Geometry: final body of the model. Coordinates: model frame, mm. Give positions to 0.01 mm unless a question says otherwise; leave off trailing zeros. Loops run counter-clockwise (first coordinate to the right, second up) from the corner with the lowest first, then second, coordinate; pieces in that order, holes last. Notation, with made-up numbers: (63.5, 65.5) - (91.5, 65.5) arc R26 cw to (91.5, 104.5) - close; hole circle Ø10 at (-3.75, 21.25). An arc over 180 degrees is marked (long way). Answer in a Markdown table with one row per item.
from build123d import *

# Parameters (mm, degrees)
F0_R     = 1.65
F0_R_2   = 2.55
F0_W     = 5
F0_H     = 10
F0_R_3   = 1.5
F0_R_4   = 3.555
F1_DEPTH = 4.75
F2_R     = 1
F3_DEPTH = 20
F4_R     = 3.555
F4_R_2   = 2.55
F5_DEPTH = 4.75


# Not quite as in the source:
# - ends of sketch curves that miss each other by under 0.0002 mm in the source are joined


with BuildPart() as f1:
    # F0 (on Top) → F1 (new body)
    with BuildSketch(Plane.XY):
        with BuildLine():
            Line((-47.640397, 42.115595), (-100.031737, 108.050449))
            ThreePointArc((-100.031737, 108.050449), (-107.8442155419, 109.1246397394), (-109.2715048598, 101.368896092))
            Line((-109.2715048598, 101.368896092), (-54.999977, 18.664241))
            Line((-54.999977, 18.664241), (-54.999977, -18.664242))
            Line((-54.999977, -18.664242), (-109.271505, -101.368897))
            ThreePointArc((-109.271505, -101.368897), (-107.8441644553, -109.1246766812), (-100.031658534, -108.0503513703))
            Line((-100.031658534, -108.0503513703), (-47.643302, -42.116283))
            ThreePointArc((-47.643302, -42.116283), (-33.7130803066, -30.9767526972), (-16.325566, -27))
            Line((-16.325566, -27), (16.325565, -27))
            ThreePointArc((16.325565, -27), (33.7130793066, -30.9767526972), (47.6433013924, -42.1162826882))
            Line((47.6433013924, -42.1162826882), (100.031658, -108.050351))
            ThreePointArc((100.031658, -108.050351), (107.8441644255, -109.1246767027), (109.2715050175, -101.3688963323))
            Line((109.2715050175, -101.3688963323), (54.999976, -18.664242))
            Line((54.999976, -18.664242), (54.999976, 18.664241))
            Line((54.999976, 18.664241), (109.271504, 101.368896))
            ThreePointArc((109.271504, 101.368896), (107.8442155121, 109.1246397609), (100.0317360662, 108.0504489474))
            Line((100.0317360662, 108.0504489474), (47.640396, 42.115595))
            ThreePointArc((47.640396, 42.115595), (33.7103248028, 30.9765618002), (16.323206, 27))
            Line((16.323206, 27), (-16.323206, 27))
            ThreePointArc((-16.323206, 27), (-33.710325083, 30.9765619354), (-47.640397, 42.115595))
        make_face()
        with Locations((-104.5, -104.5)):
            Circle(F0_R, mode=Mode.SUBTRACT)
        with Locations((-44.444977, -20.807752)):
            Circle(F0_R_2, mode=Mode.SUBTRACT)
        with Locations((-49.499977, 0)):
            Rectangle(F0_W, F0_H, mode=Mode.SUBTRACT)
        with BuildLine():
            Line((-19.581953, -16.373154), (-39.803759, -2.743263))
            ThreePointArc((-39.803759, -2.743263), (-40.6136447533, -1.8442487652), (-40.906473, -0.670199))
            Line((-40.906473, -0.670199), (-40.906473, 0.670176))
            ThreePointArc((-40.906473, 0.670176), (-40.6136450793, 1.8442251525), (-39.8037598701, 2.7432388072))
            Line((-39.8037598701, 2.7432388072), (-19.581955, 16.373149))
            ThreePointArc((-19.581955, 16.373149), (-17.0106188475, 16.5072580793), (-15.684668, 14.300086))
            Line((-15.684668, 14.300086), (-15.684668, -14.30009))
            ThreePointArc((-15.684668, -14.30009), (-17.0106178687, -16.5072615586), (-19.581953, -16.373154))
        make_face(mode=Mode.SUBTRACT)
        with Locations((-10, -10)):
            Circle(F0_R_3, mode=Mode.SUBTRACT)
        with Locations((104.5, -104.5)):
            Circle(F0_R, mode=Mode.SUBTRACT)
        with Locations((10, -10)):
            Circle(F0_R_3, mode=Mode.SUBTRACT)
        with Locations((44.444976, -20.807752)):
            Circle(F0_R_2, mode=Mode.SUBTRACT)
        with BuildLine():
            Line((19.581954, 16.373149), (39.803759, 2.743239))
            ThreePointArc((39.803759, 2.743239), (40.6136440793, 1.8442251525), (40.906472, 0.670176))
            Line((40.906472, 0.670176), (40.906472, -0.670199))
            ThreePointArc((40.906472, -0.670199), (40.6136437533, -1.8442487652), (39.803757719, -2.7432625831))
            Line((39.803757719, -2.7432625831), (19.581952, -16.373154))
            ThreePointArc((19.581952, -16.373154), (17.0106168687, -16.5072615586), (15.684667, -14.30009))
            Line((15.684667, -14.30009), (15.684667, 14.300086))
            ThreePointArc((15.684667, 14.300086), (17.0106178475, 16.5072580793), (19.581954, 16.373149))
        make_face(mode=Mode.SUBTRACT)
        with Locations((49.499976, 0)):
            Rectangle(F0_W, F0_H, mode=Mode.SUBTRACT)
        with Locations((-44.444977, 20.810818)):
            Circle(F0_R_4, mode=Mode.SUBTRACT)
        with Locations((-10, 10)):
            Circle(F0_R_3, mode=Mode.SUBTRACT)
        with Locations((-104.5, 104.5)):
            Circle(F0_R, mode=Mode.SUBTRACT)
        with Locations((10, 10)):
            Circle(F0_R_3, mode=Mode.SUBTRACT)
        with Locations((44.444976, 20.810818)):
            Circle(F0_R_4, mode=Mode.SUBTRACT)
        with Locations((104.5, 104.5)):
            Circle(F0_R, mode=Mode.SUBTRACT)
    extrude(amount=F1_DEPTH)



with BuildPart() as f3:
    # F2 (on Top) → F3 (new body)
    with BuildSketch(Plane.XY):
        with Locations((-44.444977, 20.810818)):
            Circle(F2_R)
    extrude(amount=-F3_DEPTH)


with BuildPart() as f3b:
    # F2 (on Top) → F3, piece 2 (new body)
    with BuildSketch(Plane.XY):
        with Locations((44.444976, 20.810818)):
            Circle(F2_R)
    extrude(amount=-F3_DEPTH)


with BuildPart() as f3c:
    # F2 (on Top) → F3, piece 3 (new body)
    with BuildSketch(Plane.XY):
        with Locations((-44.444977, -20.807752)):
            Circle(F2_R)
    extrude(amount=-F3_DEPTH)


with BuildPart() as f3d:
    # F2 (on Top) → F3, piece 4 (new body)
    with BuildSketch(Plane.XY):
        with Locations((44.444976, -20.807752)):
            Circle(F2_R)
    extrude(amount=-F3_DEPTH)


with BuildPart() as f1_1:
    add(f1.part)

    add(f3.part)  # F5 merges F3

    add(f3b.part)  # F5 merges F3b

    add(f3c.part)  # F5 merges F3c

    add(f3d.part)  # F5 merges F3d
    # F4 (on face) → F5 (join)
    with BuildSketch(Plane.XY.offset(4.75)):
        with Locations((-44.444977, 20.810818)):
            Circle(F4_R)
        with Locations((-44.444977, -20.807752)):
            Circle(F4_R_2)
        with Locations((44.444976, 20.810818)):
            Circle(F4_R)
        with Locations((44.444976, -20.807752)):
            Circle(F4_R_2)
    extrude(amount=-F5_DEPTH)


solid = f1_1.part
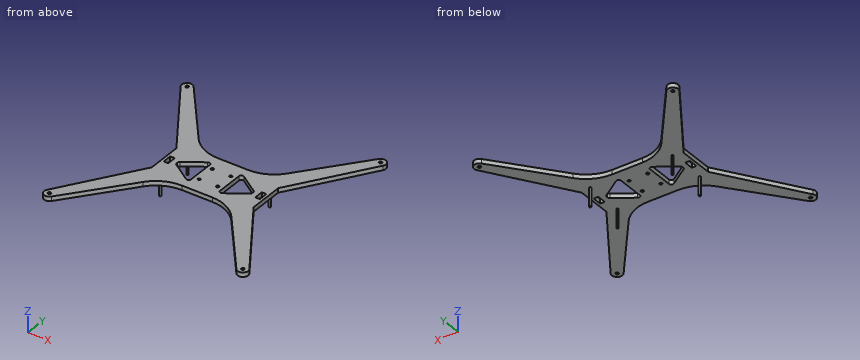
Q1. Cut plane A-A (y = 82.5). Output: boundary loops of the cut face in (x, z).
Check values:
| item | result |
|---|---|
| outline | (-96.89, 0) - (-79.73, 0) - (-79.73, 4.75) - (-96.89, 4.75) - close; (79.73, 0) - (96.89, 0) - (96.89, 4.75) - (79.73, 4.75) - close |
Q2. Cut plane D-D (x = 5). Output: boundary loops of the cut face in (y, z), and give its area (4 significant figures).
Check values:
| item | result |
|---|---|
| outline | (-27, 0) - (27, 0) - (27, 4.75) - (-27, 4.75) - close |
| area | 256.5 mm² |
Q3. Cut plane B-B (x = 68.5). Output: boundary loops of the cut face in (y, z).
Check values:
| item | result |
|---|---|
| outline | (-68.37, 0) - (-39.24, 0) - (-39.24, 4.75) - (-68.37, 4.75) - close; (39.24, 0) - (68.37, 0) - (68.37, 4.75) - (39.24, 4.75) - close |
Q4. First-contact query: pin 1 (4 mm diameter, centred on x = 104.5, y = -104.5, fed in from -Z); pin 2 (5 mm diameter, centred on y = -1.5, z = 2.5, fed in from -X); pin 3 (5 mm diameter, centred on x = -49, z = 2.5, fed in from +Y). Flat tips, straight axial feed; report the tip coordinate or a pass-through.
Check values:
| item | result |
|---|---|
| pin 1 | z = 0 |
| pin 2 | x = -55 |
| pin 3 | y = 46.97 |
Q5. Cut plane C-C (z = -15). Output: boundary loops of the cut face in (x, y).
Check values:
| item | result |
|---|---|
| outline | circle Ø2 at (-44.44, -20.81); circle Ø2 at (-44.44, 20.81); circle Ø2 at (44.44, -20.81); circle Ø2 at (44.44, 20.81) |
Q6. Material intervals for line 1 along Y through (x, z) = (10, 2.4); line 2 along Y through (x, z) = (-104.5, 1.8); line 3 along X through (y, z) = (-104.5, 2.5), sorted ascending.
Check values:
| item | result |
|---|---|
| line 1 | -27 to -11.5, -8.5 to 8.5, 11.5 to 27 |
| line 2 | -110.21 to -106.15, -102.85 to -94.1, 94.1 to 102.85, 106.15 to 110.21 |
| line 3 | -110.21 to -106.15, -102.85 to -97.21, 97.21 to 102.85, 106.15 to 110.21 |
